Source: CAD feature listing. Evaluate the final solid. Frame: model axes, mm. Coordinates: 2 decimals unless noted, no trailing zeros. Write each loop counter-clockwise with the first axis right and the second up, starting at its lowest first coordinate (ties: lowest second). Pieces come first, ordered by that corner, then holes. Notation, with made-up numbers: M -9.5,46 L 40.5,46 A16 cw 40.5,67 Z; hole C -14,-16.5 d3. An arc over 180 degrees is marked long. Answer as CSV lines item,"result". Start each with the question number.
1. Section A-A on y = 0. Return the cut outline in (x, z).
2. Section C-C on z = 4.75. Return the cut outline in (x, y), plus the area to 3 significant figures.
3. Line query: probe 1 along Y at (x, z) = (0, 2.7); probe 2 along Y at (x, z) = (-2, 8.25); probe 3 along X at (y, z) = (-3, 6.5). Output: solid intervals per line, ascending. Write a range as [from, to].
4. Section D-D on z = 3. Return the cut outline in (x, y).
5. Contact query for a flat-ended pin moving along its axis: pin 1 Ø5.5 at (x, y) = (0, 0) entering from -Z. Output: stop coordinate, or through.
```python
from build123d import *

# Parameters (mm, degrees)
BOSS_EXTRUDE1_DEPTH      = 3.5
BOSS_EXTRUDE1_DEPTH_BACK = 3.5
SKETCH1_W                = 15
SKETCH1_H                = 15
SKETCH1_R                = 3.5
FILLET1_R                = 4
FILLET2_R                = 1


with BuildPart() as part:
    # Sketch1 → Boss-Extrude1 (new, two sides: drawn at the far end of the back side and taken through both)
    with BuildSketch(Plane.XY.offset(5).offset(-BOSS_EXTRUDE1_DEPTH_BACK)):
        Rectangle(SKETCH1_W, SKETCH1_H)
        with Locations(Location((0, 0, 0), (0, 0, 180))):
            Circle(SKETCH1_R, mode=Mode.SUBTRACT)
    extrude(amount=BOSS_EXTRUDE1_DEPTH + BOSS_EXTRUDE1_DEPTH_BACK)

    # Sketch2 → Cut-Revolve1 (revolve, cut)
    with BuildSketch(Plane(origin=(0, 0, 0), x_dir=(1, 0, 0), z_dir=(0, 1, 0)), mode=Mode.PRIVATE) as cut_revolve1_sk:
        with BuildLine():
            Line((3.5, -2.770089688), (3.5, -7.229910312))
            ThreePointArc((3.5, -7.229910312), (4.15, -5), (3.5, -2.770089688))
        make_face()
    revolve(cut_revolve1_sk.sketch.rotate(Axis((0, 0, 1.5), (0, 0, 1)), 180), axis=Axis((0, 0, 1.5), (0, 0, 1)), mode=Mode.SUBTRACT)

    # Fillet1
    fillet1_edges = [part.edges().sort_by_distance(p)[0] for p in [
        (-7.5, 7.5, 5),
        (7.5, 7.5, 5),
        (7.5, -7.5, 5),
        (-7.5, -7.5, 5),
    ]]
    fillet(fillet1_edges, radius=FILLET1_R)

    # Fillet2
    fillet2_edges = [part.edges().sort_by_distance(p)[0] for p in [
        (3.5, 0, 8.5),
        (3.5, 0, 1.5),
        (7.5, 0, 1.5),
        (7.5, 0, 8.5),
        (-7.5, 0, 1.5),
        (0, 7.5, 1.5),
        (0, -7.5, 1.5),
        (-6.328427125, -6.328427125, 1.5),
        (-6.328427125, 6.328427125, 1.5),
        (6.328427125, 6.328427125, 1.5),
        (6.328427125, -6.328427125, 1.5),
        (0, -7.5, 8.5),
        (-7.5, 0, 8.5),
        (0, 7.5, 8.5),
        (-6.328427125, -6.328427125, 8.5),
        (-6.328427125, 6.328427125, 8.5),
        (6.328427125, 6.328427125, 8.5),
        (6.328427125, -6.328427125, 8.5),
    ]]
    fillet(fillet2_edges, radius=FILLET2_R)


solid = part.part
```
Values:
1,outline,"M -7.5,2.5 A1 ccw -6.5,1.5 L -4.5,1.5 A1 ccw -3.5,2.5 L -3.5,2.77 A4.15 cw -3.5,7.23 L -3.5,7.5 A1 ccw -4.5,8.5 L -6.5,8.5 A1 ccw -7.5,7.5 Z; M 3.5,2.5 A1 ccw 4.5,1.5 L 6.5,1.5 A1 ccw 7.5,2.5 L 7.5,7.5 A1 ccw 6.5,8.5 L 4.5,8.5 A1 ccw 3.5,7.5 L 3.5,7.23 A4.15 cw 3.5,2.77 Z"
2,outline,"M -7.5,-3.5 A4 ccw -3.5,-7.5 L 3.5,-7.5 A4 ccw 7.5,-3.5 L 7.5,3.5 A4 ccw 3.5,7.5 L -3.5,7.5 A4 ccw -7.5,3.5 Z; hole C 0,0 d8.28"
2,area,"157 mm²"
3,probe 1,"[-7.5, -3.5], [3.5, 7.5]"
3,probe 2,"[-7.16, -3.28], [3.28, 7.16]"
3,probe 3,"[-7.5, -2.44], [2.44, 7.5]"
4,outline,"M -7.5,-3.5 A4 ccw -3.5,-7.5 L 3.5,-7.5 A4 ccw 7.5,-3.5 L 7.5,3.5 A4 ccw 3.5,7.5 L -3.5,7.5 A4 ccw -7.5,3.5 Z; hole C 0,0 d7.27"
5,pin 1,"through"
